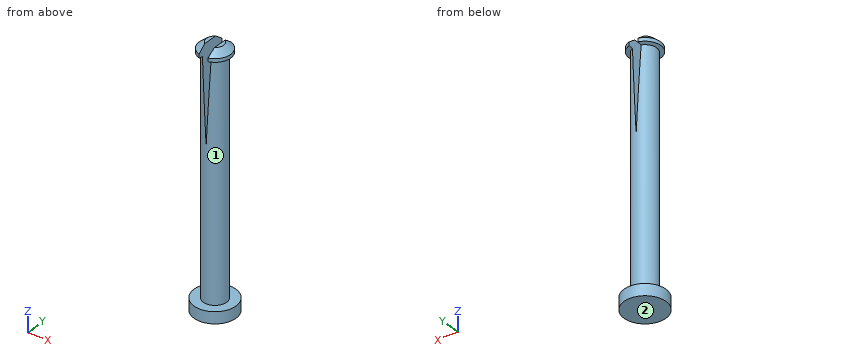
from build123d import *

# Parameters (mm, degrees)
F3_DEPTH      = 4
F3_DEPTH_BACK = 4


with BuildPart() as f2:
    # F0 (on Front) → F2 (revolve)
    with BuildSketch(Plane.XZ):
        Polygon((0, 43.75), (-1.47658, 43.75), (-2.7, 42.723429), (-2.7, 42.123429), (-2, 42), (-2, 2), (-3.6, 2), (-3.6, 0), (0, 0), align=None)
    revolve(axis=Axis((0, 0, -1.246396), (0, 0, -1)))


with BuildPart() as f3:
    # F1 (on Front) → F3 (new body, two sides)
    with BuildSketch(Plane.XZ) as f3_sk:
        Polygon((0.84, 43.75), (-0.84, 43.75), (0, 27.75), align=None)
    extrude(amount=F3_DEPTH)
    extrude(f3_sk.sketch, amount=-F3_DEPTH_BACK)


with BuildPart() as f2_1:
    add(f2.part)

    # F4: cut F3
    add(f3.part, mode=Mode.SUBTRACT)


solid = f2_1.part
Check sheet for the modelled part. Datum: model origin and axes. Units: mm. Face numbers are marked on the shaded views. Round coordinates to 2 decimals unless told otherwise and drop trailing zeros. Loops run counter-clockwise (first coordinate to the right, second up) from the corner with the lowest first, then second, coordinate; pieces in that order, holes last.
1. Sectioned sample at D-D on y = 3. Record the boundary of the cut face in (x, z), and give its area (3 significant figures).
2. Sectioned sample at C-C on z = 35. Record the boundary of the cut face in (x, y).
3. Mould release check, pull along X, two halves, no side actions. Record for the marked faces 1 and 2: released by +X, released by -X, zero draft, split by the parting line, or undercut.
4. Sectioned sample at A-A on y = 0. Record the boundary of the cut face in (x, z).
5. Gauge pin test, flat ends, axial feed: pin 1 Ø1 at (y, z) = (-2, 37) entering from +X; pin 2 Ø1.5 at (x, z) = (-1.5, 30.5) entering from +Y; pin 3 Ø3 at (y, z) = (2, 18.5) entering from -X. Record the tip position at first contact, or that the pin passes through.
6. Sectioned sample at B-B on z = 9.5. Record the boundary of the cut face in (x, y), and give its area (3 significant figures).
7. Scan lines: probe 1 along Z at (x, y) = (-0.5, -2.75); probe 2 along X at (y, z) = (1, 33.5); probe 3 along Z at (x, y) = (-1.75, 1.75). Record each from-to range of solid material in increasing order.
Recorded:
1. outline: (-1.99, 0) - (1.99, 0) - (1.99, 2) - (-1.99, 2) - close
1. area: 7.96 mm2
2. outline: (-0.38, -1.96) - (-0.38, 1.96) arc R2 ccw to start; (0.38, -1.96) arc R2 ccw to (0.38, 1.96) - close
3. face 1: split by the parting line
3. face 2: zero draft
4. outline: (-3.6, 0) - (3.6, 0) - (3.6, 2) - (2, 2) - (2, 42) - (2.7, 42.12) - (2.7, 42.72) - (1.48, 43.75) - (0.84, 43.75) - (0, 27.75) - (-0.84, 43.75) - (-1.48, 43.75) - (-2.7, 42.72) - (-2.7, 42.12) - (-2, 42) - (-2, 2) - (-3.6, 2) - close
5. pin 1: stops at x = 1.32
5. pin 2: stops at y = 1.85
5. pin 3: stops at x = -1.94
6. outline: circle Ø4 at (0, 0)
6. area: 12.6 mm2
7. probe 1: z = 0 to 2
7. probe 2: x = -1.73 to -0.3, 0.3 to 1.73
7. probe 3: z = 0 to 2, 42.08 to 42.91
